Input: dimensioned drawing with shaded views. Units: mm. Origin: part minimum x, y, z. Give positions to 0.01 mm unless a question says otherwise; leave off trailing zeros. Order: outer loops, then holes, each group sorted by start corner. A loop starts at its lowest first (then second) coordinate and runs counter-clockwise, first axis right, second up. Notation, with made-up numbers: (35, -29.75) - (75, -29.75) arc R21 ccw to (75, -22.75) - close; hole circle Ø7 at (23, -32). An arc over 180 degrees is marked (long way). Use a Markdown table: item, result.
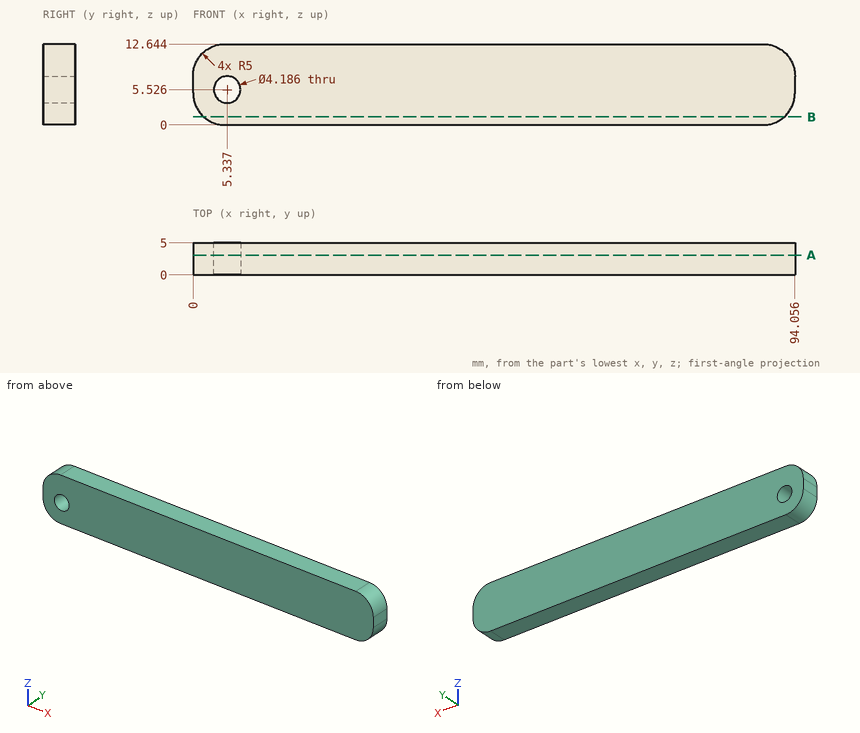
1. Material intervals for line 1 along X through (y, z) = (2.2, 3.75) (1 decimal); line 2 along X through (y, z) = (4.6, 6) (1 decimal); line 3 along X through (y, z) = (3.75, 7.75) (1 decimal), sorted ascending.
Response:
| item | result |
|---|---|
| line 1 | x = 0.2 to 4.2, 6.4 to 93.9 |
| line 2 | x = 0 to 3.3, 7.4 to 94.1 |
| line 3 | x = 0 to 94.1 |
2. Section query A-A (y = 3.1). Return loops of the section in (x, z) (1 decimal), then the cut area to 3 significant figures.
Response:
| item | result |
|---|---|
| outline | (0, 5) arc R5 ccw to (5, 0) - (89.1, 0) arc R5 ccw to (94.1, 5) - (94.1, 7.6) arc R5 ccw to (89.1, 12.6) - (5, 12.6) arc R5 ccw to (0, 7.6) - close; hole circle Ø4.2 at (5.3, 5.5) |
| area | 1,150 mm^2 |
3. Section query B-B (z = 1.25). Return loops of the section in (x, y).
Response:
| item | result |
|---|---|
| outline | (1.69, 0) - (92.36, 0) - (92.36, 5) - (1.69, 5) - close |
4. Pin query (flat end, axial travel): pin 1 (1 mm diameter, centred on y = 2.5, z = 10, fed in from -X). Return the tip coordinate at first contact, or that it passes through.
Response:
| item | result |
|---|---|
| pin 1 | stops at x = 0.36 |
